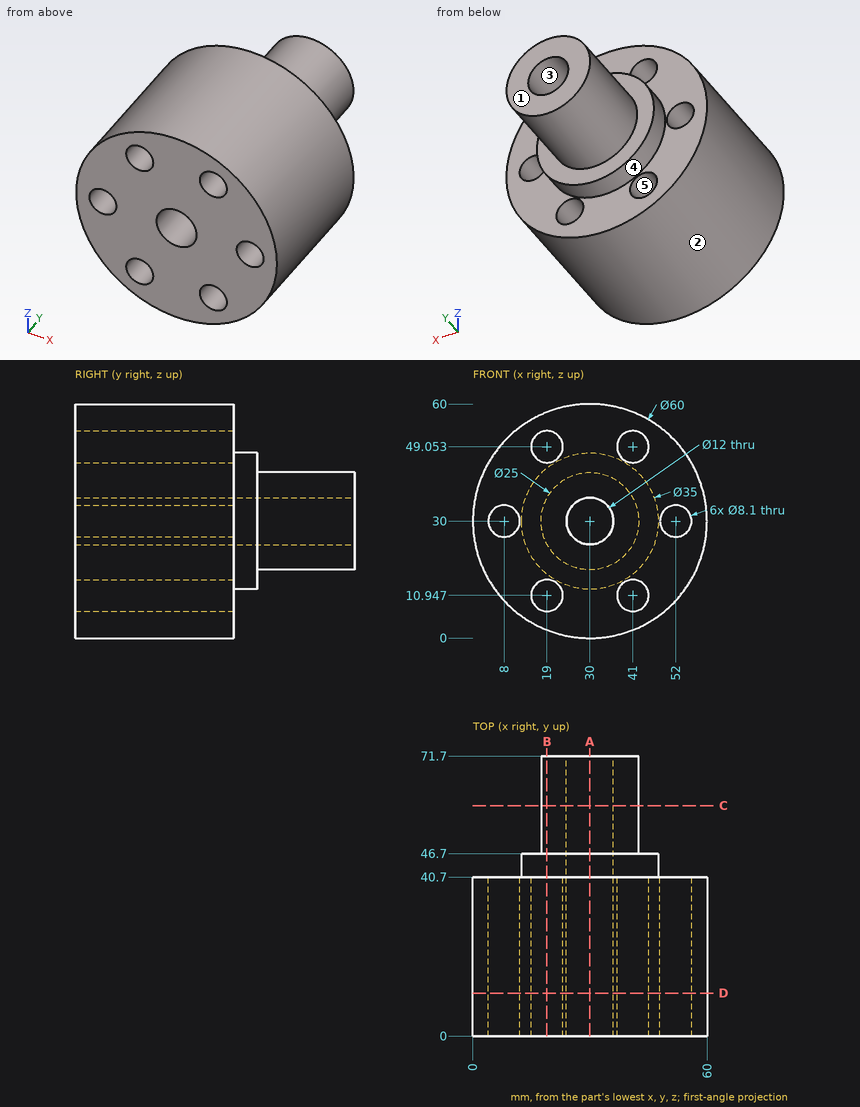
Input: dimensioned drawing with shaded views. Units: mm. Origin: part minimum x, y, z. A direction names the side the tool comes from. Give positions to 0.01 mm unless a question says otherwise; leave off trailing zeros. Loops run counter-clockwise (first coordinate to the right, second up) from the corner with the lowest first, then second, coordinate; pieces in that order, holes last. Notation, with made-up numbers: (-3, 80) -> (9, 80) arc R23 ccw to (9, 112) -> close; hole circle Ø5 at (44.25, 76). An arc over 180 degrees is marked (long way). Use a Markdown table: item, result.
Q1. First-contact query: P1, Ø4, axis at x = 49, y = 23.5, coming from the +Z side; P2, Ø5, axis at y = 22, z = 49.5, coming from the -X side; P3, Ø8, axis at y = 43.5, z = 15.5, coming from the +X side. Flat tips, straight axial feed; report the tip coordinate or a pass-through.
Entries:
| item | result |
|---|---|
| P1 | stops at z = 54.72 |
| P2 | stops at x = 5.28 |
| P3 | stops at x = 57.65 |
Q2. Section query A-A, the plane x = 30. Return the cut outline in (y, z).
Entries:
| item | result |
|---|---|
| outline | (0, 0) -> (40.7, 0) -> (40.7, 12.5) -> (46.7, 12.5) -> (46.7, 17.5) -> (71.7, 17.5) -> (71.7, 24) -> (0, 24) -> close; (0, 36) -> (71.7, 36) -> (71.7, 42.5) -> (46.7, 42.5) -> (46.7, 47.5) -> (40.7, 47.5) -> (40.7, 60) -> (0, 60) -> close |
Q3. Section query C-C, the plane y = 59. Return the cut outline in (x, z).
Entries:
| item | result |
|---|---|
| outline | circle Ø25 at (30, 30); hole circle Ø12 at (30, 30) |
Q4. Access query for the marked faces 4 and 5. Directions: +Z, -Z, +X, -X, +Y, -Y. A direction counts if a zero-diameter tool reaches every point of the face in a straight line with its end or side. Return the directions, or none.
Entries:
| item | result |
|---|---|
| face 4 | +Y |
| face 5 | +Y, -Y |
Q5. Section query B-B, the plane x = 19. Return the cut outline in (y, z), plus the area to 3 significant figures.
Entries:
| item | result |
|---|---|
| outline | (0, 2.09) -> (40.7, 2.09) -> (40.7, 6.9) -> (0, 6.9) -> close; (0, 15) -> (40.7, 15) -> (40.7, 16.39) -> (46.7, 16.39) -> (46.7, 24.06) -> (71.7, 24.06) -> (71.7, 35.94) -> (46.7, 35.94) -> (46.7, 43.61) -> (40.7, 43.61) -> (40.7, 45) -> (0, 45) -> close; (0, 53.1) -> (40.7, 53.1) -> (40.7, 57.91) -> (0, 57.91) -> close |
| area | 2,070 mm² |
Q6. Ray query, probe 1 along Z at (x, y) = (41, 9); probe 2 along X at (y, z) = (17.5, 8.5) (1 decimal); probe 3 along Z at (x, y) = (30, 56). Return the intervals inside material, ascending. Write a range as from..to.
Entries:
| item | result |
|---|---|
| probe 1 | z = 2.09..6.9, 15..45, 53.1..57.91 |
| probe 2 | x = 9.1..15.8, 22.2..37.8, 44.2..50.9 |
| probe 3 | z = 17.5..24, 36..42.5 |
Q7. Pull-direction query (X, two-part tool) for the marked faces 1, 2 and 3; classes: pulls with the +X half, pulls with the -X half, needs draft (parallel to the pull), parting line crosses it, or undercut.
Entries:
| item | result |
|---|---|
| face 1 | needs draft |
| face 2 | parting line crosses it |
| face 3 | undercut |
Q8. Section query D-D, the plane y = 11. Return the cut outline in (x, z).
Entries:
| item | result |
|---|---|
| outline | circle Ø60 at (30, 30); hole circle Ø8.1 at (8, 30); hole circle Ø8.1 at (19, 10.95); hole circle Ø8.1 at (19, 49.05); hole circle Ø12 at (30, 30); hole circle Ø8.1 at (41, 10.95); hole circle Ø8.1 at (41, 49.05); hole circle Ø8.1 at (52, 30) |
